Source: CAD feature listing. Evaluate the final solid. Frame: model axes, mm. Give positions to 0.01 mm unless a question says otherwise; leave off trailing zeros. Write each loop counter-clockwise with the first axis right and the second up, starting at its lowest first coordinate (ties: lowest second). Pieces come first, ordered by that corner, then holes. Notation, with made-up numbers: (-35.5, 63) -> (12.5, 63) arc R37 ccw to (12.5, 100) -> close; hole circle Ø3 at (10.5, 47). An arc over 180 degrees is marked (long way). Use a Markdown table: item, result. Add a question column.
```python
from build123d import *

# Parameters (mm, degrees)
EXTRUDE1_DEPTH = 6.35


with BuildPart() as part:
    # Sketch1 → Extrude1 (new body)
    with BuildSketch(Plane.XY):
        with BuildLine():
            Line((-155, -77.5), (155, -77.5))
            Line((155, -77.5), (155, -73.5))
            Line((155, -73.5), (175, -73.5))
            Line((175, -73.5), (175, -77.5))
            Line((175, -77.5), (195, -77.5))
            Line((195, -77.5), (165, 77.5))
            Line((165, 77.5), (145, 77.5))
            ThreePointArc((145, 77.5), (140, 72.5), (135, 77.5))
            Line((135, 77.5), (-135, 77.5))
            ThreePointArc((-135, 77.5), (-140, 72.5), (-145, 77.5))
            Line((-145, 77.5), (-165, 77.5))
            Line((-165, 77.5), (-195, -77.5))
            Line((-195, -77.5), (-175, -77.5))
            Line((-175, -77.5), (-175, -73.5))
            Line((-175, -73.5), (-155, -73.5))
            Line((-155, -73.5), (-155, -77.5))
        make_face()
        with BuildLine():
            Line((-130, 57.5), (-130, -47.790537842))
            ThreePointArc((-130, -47.790537842), (-126.609162538, -52.524520935), (-121.03576163, -50.837637143))
            Line((-121.03576163, -50.837637143), (-40.104522322, 54.4529007))
            ThreePointArc((-40.104522322, 54.4529007), (-39.583479402, 59.709581804), (-44.068760692, 62.5))
            Line((-44.068760692, 62.5), (-125, 62.5))
            ThreePointArc((-125, 62.5), (-128.535533906, 61.035533906), (-130, 57.5))
        make_face(mode=Mode.SUBTRACT)
        with BuildLine():
            Line((-104.895477678, -54.4529007), (-23.96423837, 50.837637143))
            ThreePointArc((-23.96423837, 50.837637143), (-18.390837462, 52.524520935), (-15, 47.790537842))
            Line((-15, 47.790537842), (-15, -57.5))
            ThreePointArc((-15, -57.5), (-16.464466094, -61.035533906), (-20, -62.5))
            Line((-20, -62.5), (-100.931239308, -62.5))
            ThreePointArc((-100.931239308, -62.5), (-105.416520598, -59.709581804), (-104.895477678, -54.4529007))
        make_face(mode=Mode.SUBTRACT)
        with BuildLine():
            Line((20, -62.5), (100.931239308, -62.5))
            ThreePointArc((100.931239308, -62.5), (105.416520598, -59.709581804), (104.895477678, -54.4529007))
            Line((104.895477678, -54.4529007), (23.96423837, 50.837637143))
            ThreePointArc((23.96423837, 50.837637143), (18.390837462, 52.524520935), (15, 47.790537842))
            Line((15, 47.790537842), (15, -57.5))
            ThreePointArc((15, -57.5), (16.464466094, -61.035533906), (20, -62.5))
        make_face(mode=Mode.SUBTRACT)
        with BuildLine():
            Line((44.068760692, 62.5), (125, 62.5))
            ThreePointArc((125, 62.5), (128.535533906, 61.035533906), (130, 57.5))
            Line((130, 57.5), (130, -47.790537842))
            ThreePointArc((130, -47.790537842), (126.609162538, -52.524520935), (121.03576163, -50.837637143))
            Line((121.03576163, -50.837637143), (40.104522322, 54.4529007))
            ThreePointArc((40.104522322, 54.4529007), (39.583479402, 59.709581804), (44.068760692, 62.5))
        make_face(mode=Mode.SUBTRACT)
    extrude(amount=EXTRUDE1_DEPTH)


solid = part.part
```
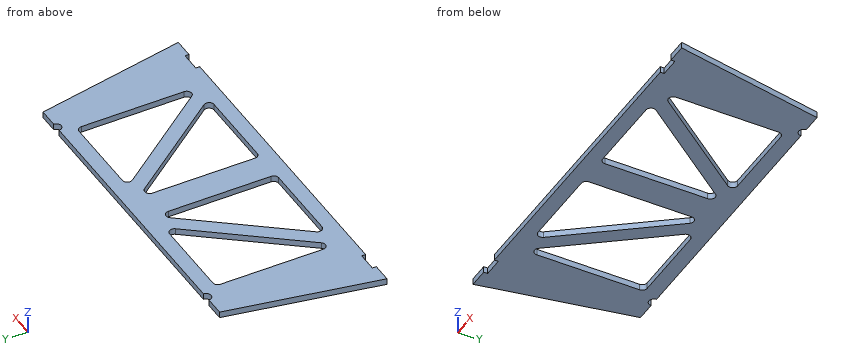
(1) Cut plane B-B on y = -36.5. Return the cut outline in (x, z).
(2) Material intervals for L1, parallel to X at y = -26, z = 4; L2, parallel to X at y = 50.5, z = 2.25; L3, parallel to Y at x = 81, z = 1, sorted ascending.
(3) Cut plane C-C on z = 4.25. Count the separate pieces of the cut face and the enclosed holes in it, then the cut area to 3 significant figures.
(4) Cut plane D-D on x = -140. Return the cut outline in (y, z), then the cut area to 4 significant figures.
(5) Cut plane A-A on x = -47.5. Return the cut outline in (y, z), then the cut area to 3 significant figures.
(6) First-contact query: pin 1 Ø4 at (x, y) = (139.5, -30.5) entering from -Z; pin 2 Ø1.9 at (x, z) = (160.5, 4.5) entering from -Y; pin 3 Ø1.2 at (y, z) = (-76, 4) entering from -X; pin 4 Ø3 at (y, z) = (10, 4.5) entering from -X. Flat tips, straight axial feed; report the tip coordinate or a pass-through.
Output:
| question | item | result |
|---|---|---|
| 1 | outline | (-187.06, 0) -> (-130, 0) -> (-130, 6.35) -> (-187.06, 6.35) -> close; (-110.02, 0) -> (-91.1, 0) -> (-91.1, 6.35) -> (-110.02, 6.35) -> close; (-15, 0) -> (15, 0) -> (15, 6.35) -> (-15, 6.35) -> close; (91.1, 0) -> (110.02, 0) -> (110.02, 6.35) -> (91.1, 6.35) -> close; (130, 0) -> (187.06, 0) -> (187.06, 6.35) -> (130, 6.35) -> close |
| 2 | L1 | -185.03 to -130, -101.94 to -83.03, -15 to 15, 83.03 to 101.94, 130 to 185.03 |
| 2 | L2 | -170.23 to -130, -43.14 to -24.22, -15.8 to 15.8, 24.22 to 43.14, 130 to 170.23 |
| 2 | L3 | -77.5 to -62.5, -23.37 to 1.25, 62.5 to 77.5 |
| 3 | separate pieces | 1 |
| 3 | enclosed holes | 4 |
| 3 | area | 31,800 mm^2 |
| 4 | outline | (-77.5, 0) -> (72.5, 0) -> (72.5, 6.35) -> (-77.5, 6.35) -> close |
| 4 | area | 952.5 mm^2 |
| 5 | outline | (-77.5, 0) -> (-62.5, 0) -> (-62.5, 6.35) -> (-77.5, 6.35) -> close; (20.22, 0) -> (44.83, 0) -> (44.83, 6.35) -> (20.22, 6.35) -> close; (62.5, 0) -> (77.5, 0) -> (77.5, 6.35) -> (62.5, 6.35) -> close |
| 5 | area | 347 mm^2 |
| 6 | pin 1 | z = 0 |
| 6 | pin 2 | y = -73.5 |
| 6 | pin 3 | x = -194.83 |
| 6 | pin 4 | x = -178.35 |
